from build123d import *

# Parameters (mm, degrees)
SKETCH1_W           = 10
SKETCH1_H           = 38
BOSS_EXTRUDE1_DEPTH = 1.5875
SKETCH2_R           = 3.45
CUT_EXTRUDE1_DEPTH  = 2.5
SKETCH3_R           = 2.875
CUT_EXTRUDE2_DEPTH  = 1.675


with BuildPart() as part:
    # Sketch1 → Boss-Extrude1 (new body, symmetric)
    with BuildSketch(Plane(origin=(0, 0, 0), x_dir=(1, 0, 0), z_dir=(0, 1, 0))):
        with BuildLine():
            ThreePointArc((-5, 19), (0, 24), (5, 19))
            Line((5, 19), (-5, 19))
        make_face()
        Rectangle(SKETCH1_W, SKETCH1_H)
        with BuildLine():
            Line((5, -19), (-5, -19))
            ThreePointArc((-5, -19), (0, -24), (5, -19))
        make_face()
    extrude(amount=BOSS_EXTRUDE1_DEPTH, both=True)

    # Sketch2 → Cut-Extrude1 (cut)
    with BuildSketch(Plane(origin=(0, 1.5875, 0), x_dir=(1, 0, 0), z_dir=(0, 1, 0))):
        with Locations((0, 19)):
            Circle(SKETCH2_R)
    extrude(amount=-CUT_EXTRUDE1_DEPTH, mode=Mode.SUBTRACT)

    # Sketch3 → Cut-Extrude2 (cut, through all)
    with BuildSketch(Plane(origin=(0, -0.9125, 0), x_dir=(1, 0, 0), z_dir=(0, 1, 0))):
        with Locations((0, 19)):
            Circle(SKETCH3_R)
    extrude(amount=-CUT_EXTRUDE2_DEPTH, mode=Mode.SUBTRACT)


solid = part.part
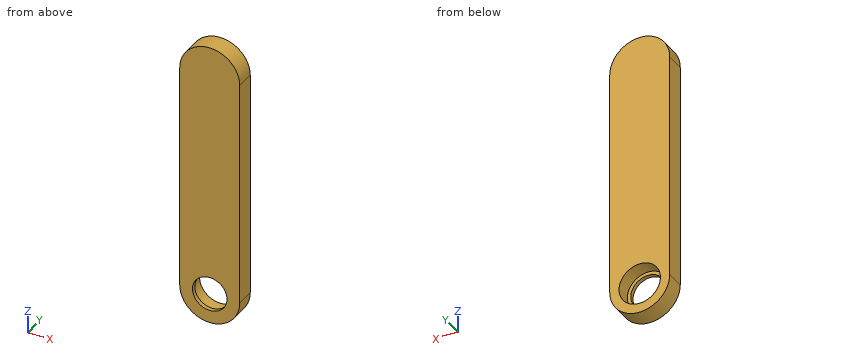
Build history of the part. All positions in model axes, mm. Give positions to 0.01 mm unless a question says otherwise; leave off trailing zeros. Write each loop counter-clockwise with the first axis right and the second up, starting at its lowest first coordinate (ties: lowest second). Pieces come first, ordered by that corner, then holes. Notation, with made-up numbers: (8, -37.5) - (37, -37.5) arc R24 cw to (37, -2.5) - close; hole circle Ø7 at (-24.75, 48.5). An arc over 180 degrees is marked (long way). Use one line per item in the form item = value. Start each with the question number.
1. Band-saw the part on A-A on y = 0.9. Write the cut outline in (x, z).
2. Band-saw the part on C-C on z = -20.5. Write the cut outline in (x, y), plus the area to 3 significant figures.
3. Band-saw the part on B-B on x = 2. Write the cut outline in (y, z), plus the area to 3 significant figures.
4. Drop a flat-ended pin along its axis: pin 1 Ø1.5 at (x, y) = (-0.5, -1) entering from +Z. Give the stop position or say it passes through.
5. Probe line 1 (X direction, y = 0.2, z = -19); line 2 (Z direction, x = 0, y = -1.4) (3 decimals); line 3 (Z direction, x = 0, y = 1.1). List the from-to ranges inside material, lowest first. Write a range as [from, to].
Conclusion:
q1.outline = (-5, -19) arc R5 ccw to (5, -19) - (5, 19) arc R5 ccw to (-5, 19) - close; hole circle Ø6.9 at (0, -19)
q2.outline = (-4.77, -1.59) - (-2.45, -1.59) - (-2.45, -0.91) - (-3.11, -0.91) - (-3.11, 1.59) - (-4.77, 1.59) - close; (2.45, -1.59) - (4.77, -1.59) - (4.77, 1.59) - (3.11, 1.59) - (3.11, -0.91) - (2.45, -0.91) - close
q2.area = 11.4 mm²
q3.outline = (-1.59, -23.58) - (1.59, -23.58) - (1.59, -21.81) - (-0.91, -21.81) - (-0.91, -21.07) - (-1.59, -21.07) - close; (-1.59, -16.93) - (-0.91, -16.93) - (-0.91, -16.19) - (1.59, -16.19) - (1.59, 23.58) - (-1.59, 23.58) - close
q3.area = 133 mm²
q4.pin_1 = 24
q5.line_1 = [-5, -3.45], [3.45, 5]
q5.line_2 = [-24, -21.875], [-16.125, 24]
q5.line_3 = [-24, -22.45], [-15.55, 24]
